Input: part model. Units: mm. Frame: model coordinates. A direction names the side the tool comes from. Coordinates: 2 decimals unless noted, no trailing zeros. Order: outer loops, then holes, each group sorted by start corner. A loop starts at its lowest first (then second) coordinate and runs counter-clockwise, first axis right, second up. Notation, with made-up numbers: M 5.25,-20 L 36.25,-20 A24 cw 36.25,-1 Z; hole C -15.75,14.5 d1. An arc over 180 degrees is marked long. Answer in a Markdown table with one row per item.
from build123d import *

# Parameters (mm, degrees)
SKETCH1_W           = 30
SKETCH1_H           = 16
BOSS_EXTRUDE1_DEPTH = 11
SHELL1_T            = 2
CUT_EXTRUDE3_REACH  = 26.779
SKETCH4_R           = 3
SKETCH4_R_2         = 2
FILLET1_R           = 1


with BuildPart() as part:
    # Sketch1 → Boss-Extrude1 (new body)
    with BuildSketch(Plane(origin=(0, 0, 0), x_dir=(1, 0, 0), z_dir=(0, 1, 0))):
        Rectangle(SKETCH1_W, SKETCH1_H)
    extrude(amount=BOSS_EXTRUDE1_DEPTH)

    # Shell1
    shell1_openings = [part.faces().sort_by_distance(p)[0] for p in [
        (15, 5.5, 0),
    ]]
    offset(amount=SHELL1_T, openings=shell1_openings, kind=Kind.INTERSECTION)

    # Cut-Extrude3: up to this face of the body (flat: up to its plane)
    cut_extrude3_end = Plane(part.part.faces().sort_by_distance((0, 0, 0))[0])
    # Sketch4 → Cut-Extrude3 (cut, up to the picked face)
    with BuildSketch(Plane(origin=(0, 13, 0), x_dir=(1, 0, 0), z_dir=(0, 1, 0)), mode=Mode.PRIVATE) as cut_extrude3_sk1:
        with Locations(Location((-12.5, -1, 0), (0, 0, 270))):
            Circle(SKETCH4_R)
    cut_extrude3_tool1 = split(extrude(cut_extrude3_sk1.sketch, amount=-CUT_EXTRUDE3_REACH, mode=Mode.PRIVATE), bisect_by=cut_extrude3_end, keep=Keep.BOTH, mode=Mode.PRIVATE)
    # Sketch4 → Cut-Extrude3 (cut, up to the picked face)
    with BuildSketch(Plane(origin=(0, 13, 0), x_dir=(1, 0, 0), z_dir=(0, 1, 0)), mode=Mode.PRIVATE) as cut_extrude3_sk2:
        with Locations(Location((-2.5, 5, 0), (0, 0, 270))):
            Circle(SKETCH4_R_2)
    cut_extrude3_tool2 = split(extrude(cut_extrude3_sk2.sketch, amount=-CUT_EXTRUDE3_REACH, mode=Mode.PRIVATE), bisect_by=cut_extrude3_end, keep=Keep.BOTH, mode=Mode.PRIVATE)
    add(cut_extrude3_tool1.solids().sort_by(Axis((-12.5, 13, 1), (0, -1, 0)))[0], mode=Mode.SUBTRACT)
    add(cut_extrude3_tool2.solids().sort_by(Axis((-2.5, 13, -5), (0, -1, 0)))[0], mode=Mode.SUBTRACT)

    # Fillet1
    fillet1_edges = [part.edges().sort_by_distance(p)[0] for p in [
        (-1, -2, 10),
        (-17, -2, 0),
        (-1, -2, -10),
        (15, -2, 0),
    ]]
    fillet(fillet1_edges, radius=FILLET1_R)


solid = part.part
1) Reachability of faces 5 (the face through (-1, 13, 0)), 6 (the face through (0, 5, 8)), 7 (the face through (-3.7, 12, -6.6)) from +Z, -Z, +X, -X, +Y, -Y: full face, straight path, thin tool, end or side. Return the list, or none.
Resolved:
| item | result |
|---|---|
| face 5 | +Z, -Z, +X, -X, +Y |
| face 6 | +X |
| face 7 | +Y |
2) Material intervals for probe 1 along Z at (x, y) = (-4.5, 0.25); probe 2 along Y at (x, z) = (12, -5.5); probe 3 along X at (y, z) = (3, -5.5), sorted ascending.
Resolved:
| item | result |
|---|---|
| probe 1 | z = -10 to -8, 8 to 10 |
| probe 2 | y = -2 to 0, 11 to 13 |
| probe 3 | x = -17 to -15 |
3) Cut plane D-D, the plane y = 1.5. Output: boundary loops of the cut face in (x, z), and give its area (3 significant figures).
Resolved:
| item | result |
|---|---|
| outline | M -17,-10 L 15,-10 L 15,-8 L -15,-8 L -15,-0.66 A3 cw -15,2.66 L -15,8 L 15,8 L 15,10 L -17,10 Z |
| area | 159 mm2 |
4) Mould query, pull axis Z, two halves, no side actions, for faces 1 (the face through (-0.776, -1.699, -9.715)), 2 (the face through (-1, 6, 10)), 3 (the face through (0, 5, -8)), 4 (the face through (15, 12, 0)). Classes: +Z half, -Z half, draft (parallel to the pull), parting line (faces both ways), or undercut.
Resolved:
| item | result |
|---|---|
| face 1 | -Z half |
| face 2 | +Z half |
| face 3 | undercut |
| face 4 | draft |
5) Cut plane B-B, the plane y = 11.75. Output: boundary loops of the cut face in (x, z).
Resolved:
| item | result |
|---|---|
| outline | M -17,-10 L 15,-10 L 15,10 L -17,10 Z; hole C -12.5,1 d6; hole C -2.5,-5 d4 |
6) Cut plane A-A, the plane z = 1. Output: boundary loops of the cut face in (x, y), and give its area (3 significant figures).
Resolved:
| item | result |
|---|---|
| outline | M -17,-1 A1 ccw -16,-2 L 14,-2 A1 ccw 15,-1 L 15,0 L -15.5,0 L -15.5,13 L -17,13 Z; M -9.5,11 L 15,11 L 15,13 L -9.5,13 Z |
| area | 132 mm2 |
7) Contact query for a flat-ended pin moving along its axis: pin 1 (1 mm diameter, centred on y = 2.5, z = 4.5, fed in from +X). Output: stop coordinate, or through.
Resolved:
| item | result |
|---|---|
| pin 1 | stops at x = -15 |
8) Cut plane C-C, the plane x = -8.5. Output: boundary loops of the cut face in (y, z), and give its area (3 significant figures).
Resolved:
| item | result |
|---|---|
| outline | M -2,-9 A1 ccw -1,-10 L 13,-10 L 13,10 L -1,10 A1 ccw -2,9 Z; hole M 0,-8 L 11,-8 L 11,8 L 0,8 Z |
| area | 124 mm2 |
